```python
from build123d import *

# Parameters (mm, degrees)
PLATE_DEPTH                    = 3
CUT_DECKPOSTS_M5_DEPTH         = 207.177108332
CUT_DECKPOSTS_M5_DEPTH_BACK    = 207.177108332
SK_DECKPOSTS_M5_R              = 2.75
CUT_LIDARRISER_M3_DEPTH        = 207.177108332
CUT_LIDARRISER_M3_DEPTH_BACK   = 207.177108332
SK_LIDARRISER_M3_R             = 1.7
CUT_LIDARCABLE_20_DEPTH        = 207.177108332
CUT_LIDARCABLE_20_DEPTH_BACK   = 207.177108332
SK_LIDARCABLE_20_R             = 10
CUT_PI5_M2P5_DEPTH             = 207.177108332
CUT_PI5_M2P5_DEPTH_BACK        = 207.177108332
SK_PI5_M2P5_R                  = 1.35
CUT_ESP32CARRIER_M3_DEPTH      = 207.177108332
CUT_ESP32CARRIER_M3_DEPTH_BACK = 207.177108332
SK_ESP32CARRIER_M3_R           = 1.7
CUT_ESTOP_22P5_DEPTH           = 207.177108332
CUT_ESTOP_22P5_DEPTH_BACK      = 207.177108332
SK_ESTOP_22P5_R                = 11.25
CUT_CAMERA_M4_DEPTH            = 207.177108332
CUT_CAMERA_M4_DEPTH_BACK       = 207.177108332
SK_CAMERA_M4_R                 = 2.25
CUT_LIGHTS_16_DEPTH            = 207.177108332
CUT_LIGHTS_16_DEPTH_BACK       = 207.177108332
SK_LIGHTS_16_R                 = 8
CUT_HANDLE_M5_DEPTH            = 207.177108332
CUT_HANDLE_M5_DEPTH_BACK       = 207.177108332
SK_HANDLE_M5_R                 = 2.75
CUT_POWERBLOCKS_M3_DEPTH       = 207.177108332
CUT_POWERBLOCKS_M3_DEPTH_BACK  = 207.177108332
SK_POWERBLOCKS_M3_R            = 1.7
CUT_K2RELAY_M2P5_DEPTH         = 207.177108332
CUT_K2RELAY_M2P5_DEPTH_BACK    = 207.177108332
SK_K2RELAY_M2P5_R              = 1.35
CUT_LIDARSPLICE_M3_DEPTH       = 207.177108332
CUT_LIDARSPLICE_M3_DEPTH_BACK  = 207.177108332
SK_LIDARSPLICE_M3_R            = 1.7
CUT_MICARRAY_M3_DEPTH          = 207.177108332
CUT_MICARRAY_M3_DEPTH_BACK     = 207.177108332
SK_MICARRAY_M3_R               = 1.7
CUT_SPEAKER_M3_DEPTH           = 207.177108332
CUT_SPEAKER_M3_DEPTH_BACK      = 207.177108332
SK_SPEAKER_M3_R                = 1.7
CUT_PASSTHROUGHS_DEPTH         = 207.177108332
CUT_PASSTHROUGHS_DEPTH_BACK    = 207.177108332


with BuildPart() as part:
    # SK_Outline → Plate (new body)
    with BuildSketch(Plane(origin=(0, 0, 0), x_dir=(1, 0, 0), z_dir=(0, 1, 0))):
        with BuildLine():
            Line((160, -110), (160, 110))
            ThreePointArc((160, 110), (154.142135624, 124.142135624), (140, 130))
            Line((140, 130), (-140, 130))
            ThreePointArc((-140, 130), (-154.142135624, 124.142135624), (-160, 110))
            Line((-160, 110), (-160, -110))
            ThreePointArc((-160, -110), (-154.142135624, -124.142135624), (-140, -130))
            Line((-140, -130), (140, -130))
            ThreePointArc((140, -130), (154.142135624, -124.142135624), (160, -110))
        make_face()
    extrude(amount=PLATE_DEPTH)

    # SK_DeckPosts_M5 → Cut_DeckPosts_M5 (cut, two sides: drawn at the far end of the back side and taken through both)
    with BuildSketch(Plane(origin=(0, 0, 0), x_dir=(1, 0, 0), z_dir=(0, 1, 0)).offset(-CUT_DECKPOSTS_M5_DEPTH_BACK)):
        with Locations(Location((140, -110, 0), (0, 0, 270))):
            Circle(SK_DECKPOSTS_M5_R)
        with Locations(Location((140, 110, 0), (0, 0, 270))):
            Circle(SK_DECKPOSTS_M5_R)
        with Locations(Location((-140, -110, 0), (0, 0, 270))):
            Circle(SK_DECKPOSTS_M5_R)
        with Locations(Location((-140, 110, 0), (0, 0, 270))):
            Circle(SK_DECKPOSTS_M5_R)
    extrude(amount=CUT_DECKPOSTS_M5_DEPTH + CUT_DECKPOSTS_M5_DEPTH_BACK, mode=Mode.SUBTRACT)

    # SK_LidarRiser_M3 → Cut_LidarRiser_M3 (cut, two sides: drawn at the far end of the back side and taken through both)
    with BuildSketch(Plane(origin=(0, 0, 0), x_dir=(1, 0, 0), z_dir=(0, 1, 0)).offset(-CUT_LIDARRISER_M3_DEPTH_BACK)):
        with Locations(Location((20, -20, 0), (0, 0, 270))):
            Circle(SK_LIDARRISER_M3_R)
        with Locations(Location((20, 20, 0), (0, 0, 270))):
            Circle(SK_LIDARRISER_M3_R)
        with Locations(Location((-20, -20, 0), (0, 0, 270))):
            Circle(SK_LIDARRISER_M3_R)
        with Locations(Location((-20, 20, 0), (0, 0, 270))):
            Circle(SK_LIDARRISER_M3_R)
    extrude(amount=CUT_LIDARRISER_M3_DEPTH + CUT_LIDARRISER_M3_DEPTH_BACK, mode=Mode.SUBTRACT)

    # SK_LidarCable_20 → Cut_LidarCable_20 (cut, two sides: drawn at the far end of the back side and taken through both)
    with BuildSketch(Plane(origin=(0, 0, 0), x_dir=(1, 0, 0), z_dir=(0, 1, 0)).offset(-CUT_LIDARCABLE_20_DEPTH_BACK)):
        with Locations(Location((0, 0, 0), (0, 0, 270))):
            Circle(SK_LIDARCABLE_20_R)
    extrude(amount=CUT_LIDARCABLE_20_DEPTH + CUT_LIDARCABLE_20_DEPTH_BACK, mode=Mode.SUBTRACT)

    # SK_Pi5_M2p5 → Cut_Pi5_M2p5 (cut, two sides: drawn at the far end of the back side and taken through both)
    with BuildSketch(Plane(origin=(0, 0, 0), x_dir=(1, 0, 0), z_dir=(0, 1, 0)).offset(-CUT_PI5_M2P5_DEPTH_BACK)):
        with Locations(Location((-97.5, 92.5, 0), (0, 0, 270))):
            Circle(SK_PI5_M2P5_R)
        with Locations(Location((-97.5, 43.5, 0), (0, 0, 270))):
            Circle(SK_PI5_M2P5_R)
        with Locations(Location((-39.5, 92.5, 0), (0, 0, 270))):
            Circle(SK_PI5_M2P5_R)
        with Locations(Location((-39.5, 43.5, 0), (0, 0, 270))):
            Circle(SK_PI5_M2P5_R)
    extrude(amount=CUT_PI5_M2P5_DEPTH + CUT_PI5_M2P5_DEPTH_BACK, mode=Mode.SUBTRACT)

    # SK_ESP32Carrier_M3 → Cut_ESP32Carrier_M3 (cut, two sides: drawn at the far end of the back side and taken through both)
    with BuildSketch(Plane(origin=(0, 0, 0), x_dir=(1, 0, 0), z_dir=(0, 1, 0)).offset(-CUT_ESP32CARRIER_M3_DEPTH_BACK)):
        with Locations(Location((-121.35, -61.5, 0), (0, 0, 270))):
            Circle(SK_ESP32CARRIER_M3_R)
        with Locations(Location((-47.65, -61.5, 0), (0, 0, 270))):
            Circle(SK_ESP32CARRIER_M3_R)
    extrude(amount=CUT_ESP32CARRIER_M3_DEPTH + CUT_ESP32CARRIER_M3_DEPTH_BACK, mode=Mode.SUBTRACT)

    # SK_EStop_22p5 → Cut_EStop_22p5 (cut, two sides: drawn at the far end of the back side and taken through both)
    with BuildSketch(Plane(origin=(0, 0, 0), x_dir=(1, 0, 0), z_dir=(0, 1, 0)).offset(-CUT_ESTOP_22P5_DEPTH_BACK)):
        with Locations(Location((-105, 0, 0), (0, 0, 270))):
            Circle(SK_ESTOP_22P5_R)
    extrude(amount=CUT_ESTOP_22P5_DEPTH + CUT_ESTOP_22P5_DEPTH_BACK, mode=Mode.SUBTRACT)

    # SK_Camera_M4 → Cut_Camera_M4 (cut, two sides: drawn at the far end of the back side and taken through both)
    with BuildSketch(Plane(origin=(0, 0, 0), x_dir=(1, 0, 0), z_dir=(0, 1, 0)).offset(-CUT_CAMERA_M4_DEPTH_BACK)):
        with Locations(Location((120, -30, 0), (0, 0, 270))):
            Circle(SK_CAMERA_M4_R)
        with Locations(Location((120, 30, 0), (0, 0, 270))):
            Circle(SK_CAMERA_M4_R)
        with Locations(Location((140, -30, 0), (0, 0, 270))):
            Circle(SK_CAMERA_M4_R)
        with Locations(Location((140, 30, 0), (0, 0, 270))):
            Circle(SK_CAMERA_M4_R)
    extrude(amount=CUT_CAMERA_M4_DEPTH + CUT_CAMERA_M4_DEPTH_BACK, mode=Mode.SUBTRACT)

    # SK_Lights_16 → Cut_Lights_16 (cut, two sides: drawn at the far end of the back side and taken through both)
    with BuildSketch(Plane(origin=(0, 0, 0), x_dir=(1, 0, 0), z_dir=(0, 1, 0)).offset(-CUT_LIGHTS_16_DEPTH_BACK)):
        with Locations(Location((130, -80, 0), (0, 0, 270))):
            Circle(SK_LIGHTS_16_R)
        with Locations(Location((130, 80, 0), (0, 0, 270))):
            Circle(SK_LIGHTS_16_R)
    extrude(amount=CUT_LIGHTS_16_DEPTH + CUT_LIGHTS_16_DEPTH_BACK, mode=Mode.SUBTRACT)

    # SK_Handle_M5 → Cut_Handle_M5 (cut, two sides: drawn at the far end of the back side and taken through both)
    with BuildSketch(Plane(origin=(0, 0, 0), x_dir=(1, 0, 0), z_dir=(0, 1, 0)).offset(-CUT_HANDLE_M5_DEPTH_BACK)):
        with Locations(Location((-151, -116, 0), (0, 0, 270))):
            Circle(SK_HANDLE_M5_R)
        with Locations(Location((-151, 116, 0), (0, 0, 270))):
            Circle(SK_HANDLE_M5_R)
    extrude(amount=CUT_HANDLE_M5_DEPTH + CUT_HANDLE_M5_DEPTH_BACK, mode=Mode.SUBTRACT)

    # SK_PowerBlocks_M3 → Cut_PowerBlocks_M3 (cut, two sides: drawn at the far end of the back side and taken through both)
    with BuildSketch(Plane(origin=(0, 0, 0), x_dir=(1, 0, 0), z_dir=(0, 1, 0)).offset(-CUT_POWERBLOCKS_M3_DEPTH_BACK)):
        with Locations(Location((-26, -84, 0), (0, 0, 270))):
            Circle(SK_POWERBLOCKS_M3_R)
        with Locations(Location((-26, -118, 0), (0, 0, 270))):
            Circle(SK_POWERBLOCKS_M3_R)
        with Locations(Location((26, -84, 0), (0, 0, 270))):
            Circle(SK_POWERBLOCKS_M3_R)
        with Locations(Location((26, -118, 0), (0, 0, 270))):
            Circle(SK_POWERBLOCKS_M3_R)
        with Locations(Location((-26, 84, 0), (0, 0, 270))):
            Circle(SK_POWERBLOCKS_M3_R)
        with Locations(Location((-26, 118, 0), (0, 0, 270))):
            Circle(SK_POWERBLOCKS_M3_R)
        with Locations(Location((26, 84, 0), (0, 0, 270))):
            Circle(SK_POWERBLOCKS_M3_R)
        with Locations(Location((26, 118, 0), (0, 0, 270))):
            Circle(SK_POWERBLOCKS_M3_R)
    extrude(amount=CUT_POWERBLOCKS_M3_DEPTH + CUT_POWERBLOCKS_M3_DEPTH_BACK, mode=Mode.SUBTRACT)

    # SK_K2Relay_M2p5 → Cut_K2Relay_M2p5 (cut, two sides: drawn at the far end of the back side and taken through both)
    with BuildSketch(Plane(origin=(0, 0, 0), x_dir=(1, 0, 0), z_dir=(0, 1, 0)).offset(-CUT_K2RELAY_M2P5_DEPTH_BACK)):
        with Locations(Location((66, -34, 0), (0, 0, 270))):
            Circle(SK_K2RELAY_M2P5_R)
        with Locations(Location((66, -51, 0), (0, 0, 270))):
            Circle(SK_K2RELAY_M2P5_R)
        with Locations(Location((101, -34, 0), (0, 0, 270))):
            Circle(SK_K2RELAY_M2P5_R)
        with Locations(Location((101, -51, 0), (0, 0, 270))):
            Circle(SK_K2RELAY_M2P5_R)
    extrude(amount=CUT_K2RELAY_M2P5_DEPTH + CUT_K2RELAY_M2P5_DEPTH_BACK, mode=Mode.SUBTRACT)

    # SK_LidarSplice_M3 → Cut_LidarSplice_M3 (cut, two sides: drawn at the far end of the back side and taken through both)
    with BuildSketch(Plane(origin=(0, 0, 0), x_dir=(1, 0, 0), z_dir=(0, 1, 0)).offset(-CUT_LIDARSPLICE_M3_DEPTH_BACK)):
        with Locations(Location((-47, 0, 0), (0, 0, 270))):
            Circle(SK_LIDARSPLICE_M3_R)
    extrude(amount=CUT_LIDARSPLICE_M3_DEPTH + CUT_LIDARSPLICE_M3_DEPTH_BACK, mode=Mode.SUBTRACT)

    # SK_MicArray_M3 → Cut_MicArray_M3 (cut, two sides: drawn at the far end of the back side and taken through both)
    with BuildSketch(Plane(origin=(0, 0, 0), x_dir=(1, 0, 0), z_dir=(0, 1, 0)).offset(-CUT_MICARRAY_M3_DEPTH_BACK)):
        with Locations(Location((91.222, 70.795, 0), (0, 0, 270))):
            Circle(SK_MICARRAY_M3_R)
        with Locations(Location((48.791, 70.783, 0), (0, 0, 270))):
            Circle(SK_MICARRAY_M3_R)
        with Locations(Location((48.787, 113.213, 0), (0, 0, 270))):
            Circle(SK_MICARRAY_M3_R)
        with Locations(Location((91.218, 113.209, 0), (0, 0, 270))):
            Circle(SK_MICARRAY_M3_R)
    extrude(amount=CUT_MICARRAY_M3_DEPTH + CUT_MICARRAY_M3_DEPTH_BACK, mode=Mode.SUBTRACT)

    # SK_Speaker_M3 → Cut_Speaker_M3 (cut, two sides: drawn at the far end of the back side and taken through both)
    with BuildSketch(Plane(origin=(0, 0, 0), x_dir=(1, 0, 0), z_dir=(0, 1, 0)).offset(-CUT_SPEAKER_M3_DEPTH_BACK)):
        with Locations(Location((95, -100, 0), (0, 0, 270))):
            Circle(SK_SPEAKER_M3_R)
        with Locations(Location((69.506, -114.726, 0), (0, 0, 270))):
            Circle(SK_SPEAKER_M3_R)
        with Locations(Location((69.503, -85.276, 0), (0, 0, 270))):
            Circle(SK_SPEAKER_M3_R)
    extrude(amount=CUT_SPEAKER_M3_DEPTH + CUT_SPEAKER_M3_DEPTH_BACK, mode=Mode.SUBTRACT)

    # SK_PassThroughs → Cut_PassThroughs (cut, two sides: drawn at the far end of the back side and taken through both)
    with BuildSketch(Plane(origin=(0, 0, 0), x_dir=(1, 0, 0), z_dir=(0, 1, 0)).offset(-CUT_PASSTHROUGHS_DEPTH_BACK)):
        with BuildLine():
            Line((-60, 118), (-40, 118))
            ThreePointArc((-40, 118), (-34, 112), (-40, 106))
            Line((-40, 106), (-60, 106))
            ThreePointArc((-60, 106), (-66, 112), (-60, 118))
        make_face()
        with BuildLine():
            Line((-60, -106), (-40, -106))
            ThreePointArc((-40, -106), (-34, -112), (-40, -118))
            Line((-40, -118), (-60, -118))
            ThreePointArc((-60, -118), (-66, -112), (-60, -106))
        make_face()
        with BuildLine():
            Line((-122, -104), (-98, -104))
            ThreePointArc((-98, -104), (-92, -110), (-98, -116))
            Line((-98, -116), (-122, -116))
            ThreePointArc((-122, -116), (-128, -110), (-122, -104))
        make_face()
        with BuildLine():
            Line((64, 30), (86, 30))
            ThreePointArc((86, 30), (92, 24), (86, 18))
            Line((86, 18), (64, 18))
            ThreePointArc((64, 18), (58, 24), (64, 30))
        make_face()
        with BuildLine():
            Line((98, -50), (98, -62))
            ThreePointArc((98, -62), (92, -68), (86, -62))
            Line((86, -62), (86, -50))
            ThreePointArc((86, -50), (92, -44), (98, -50))
        make_face()
    extrude(amount=CUT_PASSTHROUGHS_DEPTH + CUT_PASSTHROUGHS_DEPTH_BACK, mode=Mode.SUBTRACT)


solid = part.part
```
Part model, mm, in its own coordinate system. Round coordinates to 2 decimals unless told otherwise and drop trailing zeros. Loops run counter-clockwise (first coordinate to the right, second up) from the corner with the lowest first, then second, coordinate; pieces in that order, holes last.
Item 1: Cut at A-A, the plane x = 130. Give the cut face in (y, z).
Item 2: Cut at B-B, the plane x = 4. Give the cut face in (y, z).
Item 3: Drill centre lines: line 1 (Z direction, x = 120, y = 2.1); line 2 (Z direction, x = -140, y = 1.3); line 3 (X direction, y = 1.35, z = 30). Where is each one in solid material? Low to high.
Item 4: Mould opens along Z. For faces 1 (the face through (153.986, 1.479, 124.297)), 2 (the face through (-153.986, 1.479, -124.297)), 3 (the face through (122.19, 1.48, 78.27)) say: +Z half, -Z half, draft (parallel to the pull), parting line (faces both ways), or undercut.
Item 5: Cut at C-C, the plane y = 2.05. State how many separate pieces and enclosed holes the cut face has, then the cut area to 3 significant figures.
Item 6: Drop a flat-ended pin along its axis: P1, Ø4, axis at x = -47.65, z = 61.5, coming from the +Y side. Give the stop position or say it passes through.
A:
1. outline: (0, -130) - (3, -130) - (3, -88) - (0, -88) - close; (0, -72) - (3, -72) - (3, 72) - (0, 72) - close; (0, 88) - (3, 88) - (3, 130) - (0, 130) - close
2. outline: (0, -130) - (3, -130) - (3, -9.17) - (0, -9.17) - close; (0, 9.17) - (3, 9.17) - (3, 130) - (0, 130) - close
3. line 1: z = -130 to -32.25, -27.75 to 27.75, 32.25 to 130
3. line 2: z = -130 to -112.75, -107.25 to 107.25, 112.75 to 130
3. line 3: x = -160 to 117.75, 122.25 to 137.75, 142.25 to 160
4. face 1: +Z half
4. face 2: -Z half
4. face 3: undercut
5. separate pieces: 1
5. enclosed holes: 49
5. area: 79,500 mm2
6. P1: stops at y = 3
